Work out the finished part from the listing and answer in its coordinate system (mm). Face numbers are marked on the shaded views. Round coordinates to 2 decimals unless told otherwise and drop trailing zeros. Loops run counter-clockwise (first coordinate to the right, second up) from the corner with the lowest first, then second, coordinate; pieces in that order, holes last. Notation, with made-up numbers: (60.25, 66) - (105.25, 66) arc R15 cw to (105.25, 74) - close; hole circle Ø3 at (57, 47.5). An arc over 180 degrees is marked (long way). Answer as CSV lines item,"result". Start each with the question number.
Q1. Section B-B on y = -3.5 is taken. Write down the section's boundary in (x, z) (3 decimals).
Q2. The mould has two halves that part along X. Classify the marked faces 1 and 2: +X half, -X half, draft (parallel to the pull), parting line (faces both ways), or undercut.
Q3. Straight lines are drawn through the part: L1, parallel to X at y = -136, z = -20 (3 decimals); L2, parallel to Y at x = 7, z = -26.75; L3, parallel to Z at x = -7.5, y = -17.5. For each, find the intervals that lie inside material, in ascending order. Write a range as [from, to].
Q4. Section D-D on y = -129.5 is taken. Write down the section's boundary in (x, z) (3 decimals).
Q5. Section C-C on x = -5.5 is taken. Write down the section's boundary in (y, z), then the cut area to 3 significant figures.
Q6. Section A-A on z = -20 is taken. Write down the section's boundary in (x, y) (3 decimals).
Q7. Each of these flat-tipped pins is pushed along its axis until it touches: pin 1 Ø3.5 at (x, z) = (-35, -27.5) entering from +Y; pin 2 Ø5 at (y, z) = (-33, -2) entering from -X; pin 3 Ø1.6 at (y, z) = (-136, -15.5) entering from +X. Where does it stop, or does it pass through?
```python
from build123d import *

# Parameters (mm, degrees)
SKETCH1_R                = 1.75
BOSS_EXTRUDE1_DEPTH      = 1.5
BOSS_EXTRUDE2_DEPTH      = 82
BOSS_EXTRUDE3_DEPTH      = 1.5
BOSS_EXTRUDE3_DEPTH_BACK = 1.5
BOSS_EXTRUDE4_DEPTH      = 2
SKETCH5_R                = 1.75
CUT_EXTRUDE1_DEPTH       = 2
CUT_EXTRUDE2_DEPTH       = 149.716477315
CUT_EXTRUDE2_DEPTH_BACK  = 149.716477315
SKETCH6_W                = 82
SKETCH6_H                = 11.5
BOSS_EXTRUDE6_START      = -2
SKETCH7_W                = 3
SKETCH7_H                = 4
BOSS_EXTRUDE6_DEPTH      = 2.5
FILLET1_R                = 2
CHAMFER1_SIZE            = 1
FILLET2_R                = 8
SKETCH8_W                = 26
SKETCH8_H                = 23
CUT_EXTRUDE3_DEPTH       = 22.4262221


with BuildPart() as part:
    # Sketch1 → Boss-Extrude1 (new body)
    with BuildSketch(Plane.XY):
        with BuildLine():
            Line((-37.75, -134.5), (37.75, -134.5))
            Line((37.75, -134.5), (41, -134.5))
            Line((41, -134.5), (41, -132.48653227))
            ThreePointArc((41, -132.48653227), (42.775, -129.5), (41, -126.51346773))
            Line((41, -126.51346773), (41, -6.48653227))
            ThreePointArc((41, -6.48653227), (42.775, -3.5), (41, -0.51346773))
            Line((41, -0.51346773), (41, 0))
            Line((41, 0), (-41, 0))
            Line((-41, 0), (-41.072829787, -0.55426172))
            ThreePointArc((-41.072829787, -0.55426172), (-42.774743802, -3.541738254), (-41, -6.48653227))
            Line((-41, -6.48653227), (-41, -126.51346773))
            ThreePointArc((-41, -126.51346773), (-42.775, -129.5), (-41, -132.48653227))
            Line((-41, -132.48653227), (-41, -134.5))
            Line((-41, -134.5), (-37.75, -134.5))
        make_face()
        with Locations((-39.375, -129.5)):
            Circle(SKETCH1_R, mode=Mode.SUBTRACT)
        with Locations((39.375, -129.5)):
            Circle(SKETCH1_R, mode=Mode.SUBTRACT)
        with Locations((39.375, -3.5)):
            Circle(SKETCH1_R, mode=Mode.SUBTRACT)
        with Locations((-39.375, -3.5)):
            Circle(SKETCH1_R, mode=Mode.SUBTRACT)
    extrude(amount=BOSS_EXTRUDE1_DEPTH)

    # Sketch2 → Boss-Extrude2 (add)
    with BuildSketch(Plane.ZY.offset(41)):
        Polygon((1.5, -134.5), (1.5, -136.7), (-40, -136.7), (-40, -134.7), (0, -134.7), (0, -134.5), (0, -132.48653227), (1.5, -132.48653227), align=None)
    extrude(amount=-BOSS_EXTRUDE2_DEPTH)

    # Sketch3 → Boss-Extrude3 (add, two sides: drawn at the far end of the back side and taken through both)
    with BuildSketch(Plane(origin=(-15, 0, 0), x_dir=(0, 0, -1), z_dir=(1, 0, 0)).offset(-BOSS_EXTRUDE3_DEPTH_BACK)):
        Polygon((0, -119.7), (15, -134.7), (0, -134.7), align=None)
    extrude(amount=BOSS_EXTRUDE3_DEPTH + BOSS_EXTRUDE3_DEPTH_BACK)

    # Sketch4 → Boss-Extrude4 (add)
    with BuildSketch(Plane.XZ.offset(136.7)):
        with BuildLine():
            Line((-41, -17.01346773), (-41, -22.98653227))
            ThreePointArc((-41, -22.98653227), (-42.775, -20), (-41, -17.01346773))
        make_face()
        with BuildLine():
            Line((41, -17.01346773), (41, -22.98653227))
            ThreePointArc((41, -22.98653227), (42.775, -20), (41, -17.01346773))
        make_face()
    extrude(amount=-BOSS_EXTRUDE4_DEPTH)

    # Sketch5 → Cut-Extrude1 (cut)
    with BuildSketch(Plane.XZ.offset(136.7)):
        with Locations(Location((39.375, -20, 0), (0, 0, 270))):
            Circle(SKETCH5_R)
        with Locations(Location((-39.375, -20, 0), (0, 0, 270))):
            Circle(SKETCH5_R)
    extrude(amount=-CUT_EXTRUDE1_DEPTH, mode=Mode.SUBTRACT)

    # Sketch6 → Cut-Extrude2 (cut, two sides: drawn at the far end of the back side and taken through both)
    with BuildSketch(Plane.XZ.offset(136.7).offset(-CUT_EXTRUDE2_DEPTH_BACK)):
        with Locations((0, -34.25)):
            Rectangle(SKETCH6_W, SKETCH6_H)
    extrude(amount=CUT_EXTRUDE2_DEPTH + CUT_EXTRUDE2_DEPTH_BACK, mode=Mode.SUBTRACT)

    # Sketch7 → Boss-Extrude6 (add)
    with BuildSketch(Plane.XZ.offset(136.7).offset(BOSS_EXTRUDE6_START)):
        with Locations((-34.8, -26.5)):
            Rectangle(SKETCH7_W, SKETCH7_H)
        with Locations((34.8, -26.5)):
            Rectangle(SKETCH7_W, SKETCH7_H)
    extrude(amount=-BOSS_EXTRUDE6_DEPTH)

    # Fillet1
    fillet1_edges = [part.edges().sort_by_distance(p)[0] for p in [
        (41, -135.7, -28.5),
        (-41, -135.7, -28.5),
    ]]
    fillet(fillet1_edges, radius=FILLET1_R)

    # Chamfer1
    chamfer1_edges = [part.edges().sort_by_distance(p)[0] for p in [
        (-34.8, -134.7, -24.5),
        (-34.8, -132.2, -24.5),
        (34.8, -134.7, -24.5),
        (34.8, -132.2, -24.5),
    ]]
    chamfer(chamfer1_edges, length=CHAMFER1_SIZE)

    # Fillet2
    # the kernel refuses this fillet: 8 mm, written as the material it takes off along each edge
    with BuildSketch(Plane(origin=(-28.303909917, -133.2, -24.5), x_dir=(0, -1.0, -1.118394266079786e-11), z_dir=(-1, 0, 0))) as fillet2_piece_1:
        with BuildLine():
            CenterArc((4.243746579, -7.06996192), FILLET2_R, 117.902496562, 17.097503438)
            Line((-1.413107671, -1.413107671), (0, 0))
            Line((0, 0), (0.5, 0))
        make_face()
    extrude(amount=12.992180166, mode=Mode.SUBTRACT)
    with BuildSketch(Plane(origin=(28.303909917, -133.2, -24.5), x_dir=(0, 0.7071067811865501, -0.7071067811865448), z_dir=(1, 0, 0))) as fillet2_piece_2:
        with BuildLine():
            CenterArc((1.998436033, -8), FILLET2_R, 90, 17.097503438)
            Line((-0.353553391, -0.353553391), (0, 0))
            Line((0, 0), (1.998436033, 0))
        make_face()
    extrude(amount=12.992180166, mode=Mode.SUBTRACT)

    # Sketch8 → Cut-Extrude3 (cut)
    with BuildSketch(Plane.XZ.offset(136.7)):
        with Locations((4, -14)):
            Rectangle(SKETCH8_W, SKETCH8_H)
    extrude(amount=-CUT_EXTRUDE3_DEPTH, mode=Mode.SUBTRACT)


solid = part.part
```
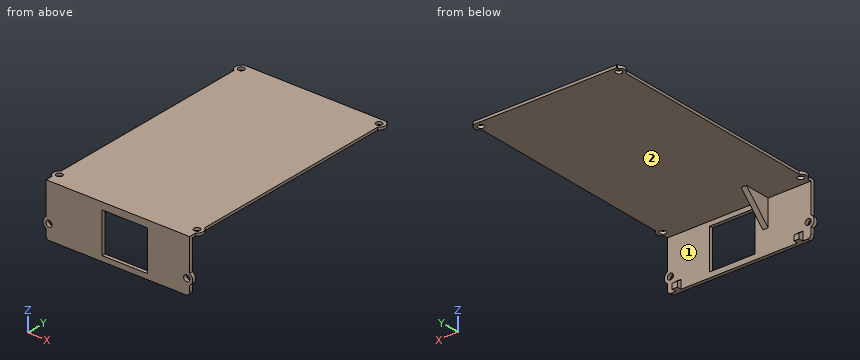
Findings:
1,outline,"(-42.775, 0) - (-41.125, 0) - (-41.125, 1.5) - (-42.775, 1.5) - close; (-37.625, 0) - (37.625, 0) - (37.625, 1.5) - (-37.625, 1.5) - close; (41.125, 0) - (42.775, 0) - (42.775, 1.5) - (41.125, 1.5) - close"
2,face 1,"undercut"
2,face 2,"draft"
3,L1,"x = [-42.775, -41.125], [-37.625, -9], [17, 37.625], [41.125, 42.775]"
3,L2,"y = [-136.7, -134.7]"
3,L3,"z = [0, 1.5]"
4,outline,"(-42.775, 0) - (-41.125, 0) - (-41.125, 1.5) - (-42.775, 1.5) - close; (-37.625, 0) - (-16.5, 0) - (-16.5, -9.8) - (-13.5, -9.8) - (-13.5, 0) - (37.625, 0) - (37.625, 1.5) - (-37.625, 1.5) - close; (41.125, 0) - (42.775, 0) - (42.775, 1.5) - (41.125, 1.5) - close"
5,outline,"(-136.7, -28.5) - (-134.7, -28.5) - (-134.7, -25.5) - (-136.7, -25.5) - close; (-136.7, -2.5) - (-134.7, -2.5) - (-134.7, 0) - (0, 0) - (0, 1.5) - (-136.7, 1.5) - close"
5,area,"216 mm^2"
6,outline,"(-42.775, -136.7) - (-41.125, -136.7) - (-41.125, -134.7) - (-42.775, -134.7) - close; (-37.625, -136.7) - (-9, -136.7) - (-9, -134.7) - (-37.625, -134.7) - close; (17, -136.7) - (37.625, -136.7) - (37.625, -134.7) - (17, -134.7) - close; (41.125, -136.7) - (42.775, -136.7) - (42.775, -134.7) - (41.125, -134.7) - close"
7,pin 1,"stops at y = -132.2"
7,pin 2,"stops at x = -41"
7,pin 3,"stops at x = 41"
